Geometry: final body of the model. Coordinates: model frame, mm. A direction names the side the tool comes from. Give positions to 0.01 mm unless a question says otherwise; leave off trailing zeros. Write each loop counter-clockwise with the first axis right and the second up, starting at its lowest first coordinate (ties: lowest second). Pieces come first, ordered by that corner, then holes. Notation, with made-up numbers: (-11.75, 19.5) -> (41.25, 19.5) arc R24 cw to (41.25, 56.5) -> close; hole circle Ø3 at (6.5, 11). An arc over 180 degrees is marked (long way). Answer in a Markdown table with one row per item. Add a question column.
Item 1: Material intervals for probe 1 along Z at (x, y) = (644.5, 0); probe 2 along X at (y, z) = (2.5, -1.5); probe 3 along Y at (x, z) = (347, 0.75), sorted ascending. Write a range as from..to.
Item 2: Section query A-A on z = 0. Output: boundary loops of the cut face in (x, y), plus the area to 3 significant figures.
Item 3: Draft query along Y for faces 3 (the cylindrical face through (650.67, -1.08, -4.88)), 4 (the cylindrical face through (326.86, -2.17, -9.76)), 5 (the flat face through (663, -5, -2)). Return one class per face: +Y half, -Y half, draft (parallel to the pull), parting line (faces both ways), or undercut.
Item 4: Section query B-B on y = 1.5. Output: boundary loops of the cut face in (x, z), plus the area to 3 significant figures.
Item 5: First-contact query: P1, Ø8, axis at x = 548, y = -6, coming from the -Z side; P2, Ø2, axis at y = -8, z = 8, coming from the +X side; P3, Ø1, axis at x = 350.5, y = 5, coming from the +Z side; P4, Ø4, axis at x = 76.5, z = 3, coming from the +Y side. Flat tips, straight axial feed; report the tip coordinate or a pass-through.
Item 6: Access query for faces 1 (the flat face through (0, 0, 0)), 2 (the flat face through (638, 0, 0)). Directions: +Z, -Z, +X, -X, +Y, -Y. A direction counts if a zero-diameter tool reaches every point of the face in a straight line with its end or side. Return the directions, or none.
Item 7: Section query C-C on x = 605. Output: boundary loops of the cut face in (y, z), plus the area to 3 significant figures.
```python
from build123d import *

# Parameters (mm, degrees)
F0_R      = 10
F1_DEPTH  = 638
F1_FACE_R = 10
F2_DEPTH  = 25
F3_R      = 5
F4_DEPTH  = 25


with BuildPart() as f1:
    # F0 (on Right) → F1 (new body)
    with BuildSketch(Plane.YZ):
        Circle(F0_R)
    extrude(amount=F1_DEPTH)

    # F1_face (on face) → F2 (join)
    with BuildSketch(Plane.YZ.offset(638)):
        Circle(F1_FACE_R)
    extrude(amount=F2_DEPTH)

    # F3 (on face) → F4 (cut)
    with BuildSketch(Plane.YZ.offset(663)):
        Circle(F3_R)
    extrude(amount=-F4_DEPTH, mode=Mode.SUBTRACT)


solid = f1.part
```
Findings below:
| question | item | result |
|---|---|---|
| 1 | probe 1 | z = -10..-5, 5..10 |
| 1 | probe 2 | x = 0..638 |
| 1 | probe 3 | y = -9.97..9.97 |
| 2 | outline | (0, -10) -> (663, -10) -> (663, -5) -> (638, -5) -> (638, 5) -> (663, 5) -> (663, 10) -> (0, 10) -> close |
| 2 | area | 13,000 mm^2 |
| 3 | face 3 | undercut |
| 3 | face 4 | parting line |
| 3 | face 5 | draft |
| 4 | outline | (0, -9.89) -> (663, -9.89) -> (663, -4.77) -> (638, -4.77) -> (638, 4.77) -> (663, 4.77) -> (663, 9.89) -> (0, 9.89) -> close |
| 4 | area | 12,900 mm^2 |
| 5 | P1 | stops at z = -9.8 |
| 5 | P2 | passes through |
| 5 | P3 | stops at z = 8.93 |
| 5 | P4 | stops at y = 9.95 |
| 6 | face 1 | +Z, -Z, -X, +Y, -Y |
| 6 | face 2 | +X |
| 7 | outline | circle Ø20 at (0, 0) |
| 7 | area | 314 mm^2 |
